Could you check a few things on this model? Use its own coordinates, in mm. A direction names the side the tool comes from. Coordinates: 2 decimals unless noted, no trailing zeros. Loops run counter-clockwise (first coordinate to the right, second up) from the corner with the lowest first, then second, coordinate; pieces in that order, holes last.
1) Imagine slicing it at A-A on y = 47. Please give me the cut outline in (x, z).
2) If I drill on line 1 along Z through (x, y) = (34, 70); line 2 along Y through (x, z) = (52.5, -42.5); line 3 along X through (y, z) = (71, 49.5), over which ranges is the centre line in solid material (lowest first)?
3) Imagine slicing it at C-C on x = 120.5. Please give me the cut outline in (y, z), plus the area to 3 significant figures.
4) Will these pins go through, and if not, where does the flat tip stop? P1, Ø1.5, axis at y = 38, z = 12, coming from the +X side (3 decimals); P2, Ø8, axis at y = 8.5, z = -38.5, coming from the +X side; P3, Ø4, axis at x = 63.5, z = 11, coming from the +Y side.
5) Imagine slicing it at B-B on z = -50.5. Please give me the cut outline in (x, y).
6) Thinking about a two-plate mould opening in X: for faces 4 (the face through (59, 37, 63)), 5 (the face through (77, 0, 1)), 6 (the face through (138.954, 36.975, 0.882)), which applies, released by +X, released by -X, zero draft, split by the parting line, or undercut?
7) Imagine slicing it at D-D on x = 94.5. Please give me the cut outline in (y, z), plus the area to 3 significant figures.
8) For faces 1 (the face through (0, 37, 1)), 2 (the face through (115, 75, 0)), 3 (the face through (134.9, 38, 0.8)), which set-ups out of +Z, -Z, +X, -X, +Y, -Y let a thin tool reach every point of the face, with its end or its side?
```python
from build123d import *

# Parameters (mm, degrees)
SKETCH2_W           = 3
SKETCH2_H           = 75
SKETCH2_W_2         = 163.301270189
SKETCH2_H_2         = 3
BOSS_EXTRUDE3_DEPTH = 60
BOSS_EXTRUDE4_START = 60
SKETCH2_3_W         = 163.301270189
SKETCH2_3_H         = 3
SKETCH2_3_W_2       = 3
SKETCH2_3_H_2       = 75
BOSS_EXTRUDE4_DEPTH = 3


with BuildPart() as part:
    # Sketch2 → Boss-Extrude3 (new body)
    with BuildSketch(Plane.XY):
        with Locations((-1.5, 37.5)):
            Rectangle(SKETCH2_W, SKETCH2_H)
        Polygon((156.837168574, 0), (160.301270189, 0), (117, 75), (113.535898385, 75), align=None)
        with Locations((78.650635095, -1.5)):
            Rectangle(SKETCH2_W_2, SKETCH2_H_2)
    extrude(amount=BOSS_EXTRUDE3_DEPTH)

    # Sketch2<3> → Boss-Extrude4 (add)
    with BuildSketch(Plane.XY.offset(BOSS_EXTRUDE4_START)):
        Polygon((156.837168574, 0), (160.301270189, 0), (117, 75), (113.535898385, 75), align=None)
        with Locations((78.650635095, -1.5)):
            Rectangle(SKETCH2_3_W, SKETCH2_3_H)
        Polygon((0, 0), (156.837168574, 0), (113.535898385, 75), (0, 75), align=None)
        with Locations((-1.5, 37.5)):
            Rectangle(SKETCH2_3_W_2, SKETCH2_3_H_2)
    extrude(amount=BOSS_EXTRUDE4_DEPTH)

    # Mirror2: part across plane


with BuildPart() as part_1:
    add(part.part)
    add(part.part.mirror(Plane.XY))


solid = part_1.part
```
Filled in:
1. outline: (-3, -63) - (133.17, -63) - (133.17, 63) - (-3, 63) - close; hole (0, -60) - (129.7, -60) - (129.7, 60) - (0, 60) - close
2. line 1: z = -63 to -60, 60 to 63
2. line 2: y = -3 to 0
2. line 3: x = -3 to 0, 115.85 to 119.31
3. outline: (-3, -63) - (68.94, -63) - (68.94, 63) - (-3, 63) - close; hole (0, -60) - (62.94, -60) - (62.94, 60) - (0, 60) - close
3. area: 1,510 mm2
4. P1: stops at x = 138.795
4. P2: stops at x = 157.7
4. P3: stops at y = 0
5. outline: (-3, -3) - (160.3, -3) - (160.3, 0) - (117, 75) - (113.54, 75) - (156.84, 0) - (0, 0) - (0, 75) - (-3, 75) - close
6. face 4: zero draft
6. face 5: undercut
6. face 6: released by +X
7. outline: (-3, -63) - (75, -63) - (75, -60) - (0, -60) - (0, 60) - (75, 60) - (75, 63) - (-3, 63) - close
7. area: 828 mm2
8. face 1: +Y
8. face 2: +Z, -Z, +X, -X, +Y
8. face 3: none
